Answer from the drawing. Dimensions are ordinates in mm from the lowest x, y and z of the part. Coordinates: 2 decimals unless noted, no trailing zeros. Order: outer loops, then holes, each group sorted by start corner. A loop starts at its lowest first (then second) coordinate and runs counter-clockwise, first axis right, second up. Notation, with made-up numbers: (28, 40.5) - (59, 40.5) arc R5 cw to (59, 47.5) - close; hole circle Ø1 at (-26.5, 27). An arc over 180 degrees is marked (long way). Use CSV: the item, a comma, the result in double quotes. Start each with the question number.
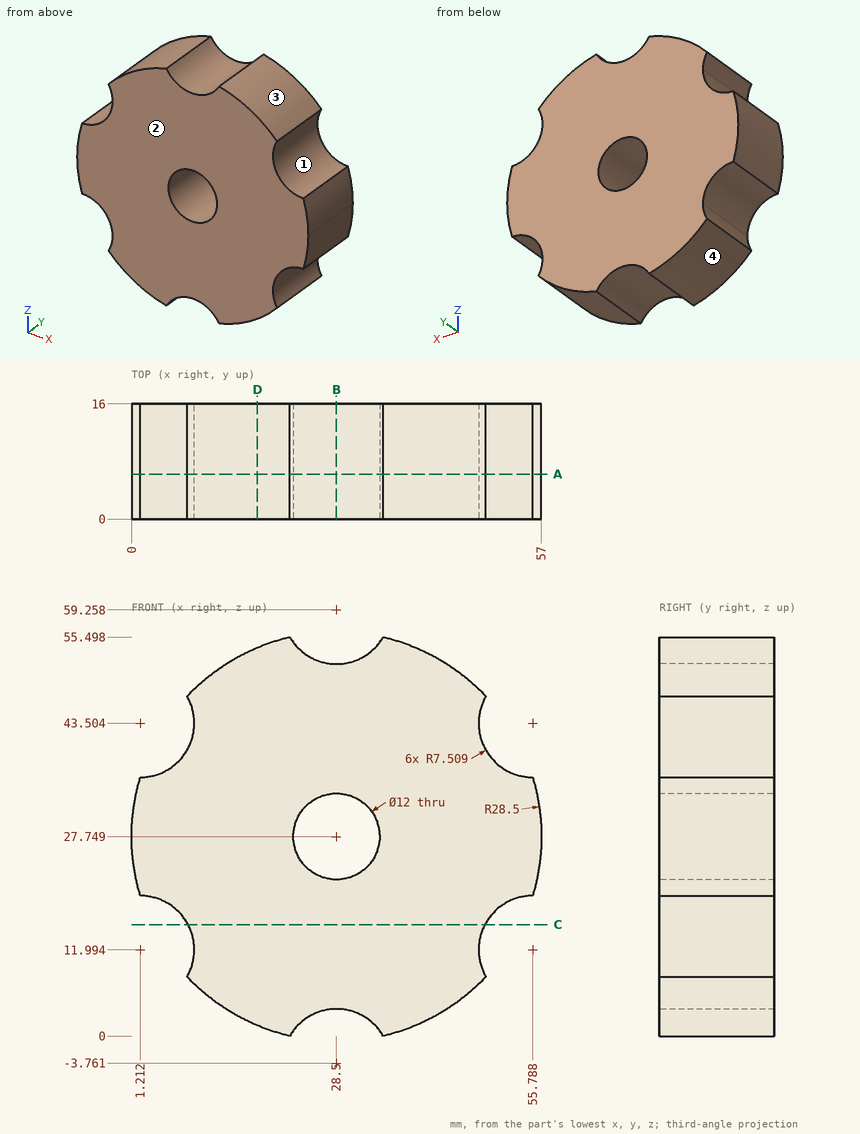
1) Straight lines are drawn through the part: line 1 (X direction, y = 10.75, z = 28) (1 decimal); line 2 (Z direction, x = 23.5, y = 13.25) (1 decimal); line 3 (X direction, y = 4.75, z = 29). For each, find the intervals that lie inside material, in ascending order. Write a range as [from, to].
2) The part is cut by section B-B on x = 28.5. Determine the outline of the cut face in (y, z).
3) The part is cut by section D-D on x = 17.5. Determine the outline of the cut face in (y, z).
4) The part is cut by section C-C on z = 15.5. Determine the outline of the cut face in (x, y), plus the area to 3 significant figures.
5) For a pull along Z with two mould halves and no side action, classify the marked faces 1, 2, 3 and 4 as +Z half, -Z half, draft (parallel to the pull), parting line (faces both ways), or undercut.
6) Flat-ended cylindrical pins translate along their axes: P1, Ø4, axis at y = 10.5, z = 11, coming from the +X side; P2, Ø1, axis at x = 37.5, y = 3.5, coming from the -Z side; P3, Ø1.5, axis at y = 12.5, z = 39, coming from the -X side. Find the tip coordinate at first contact, or state that the pin passes through.
7) The part is cut by section A-A on y = 6.25. Determine the outline of the cut face in (x, z) (1 decimal).
Answer key:
1,line 1,"[0, 22.5], [34.5, 57]"
1,line 2,"[1.8, 24.4], [31.1, 53.7]"
1,line 3,"[0.03, 22.63], [34.37, 56.97]"
2,outline,"(0, 3.75) - (16, 3.75) - (16, 21.75) - (0, 21.75) - close; (0, 33.75) - (16, 33.75) - (16, 51.75) - (0, 51.75) - close"
3,outline,"(0, 1.46) - (16, 1.46) - (16, 54.04) - (0, 54.04) - close"
4,outline,"(7.85, 0) - (49.15, 0) - (49.15, 16) - (7.85, 16) - close"
4,area,"661 mm^2"
5,face 1,"undercut"
5,face 2,"draft"
5,face 3,"+Z half"
5,face 4,"-Z half"
6,P1,"x = 48.9"
6,P2,"z = 0.55"
6,P3,"x = 6.58"
7,outline,"(1.2, 19.5) arc R7.5 cw to (7.7, 8.2) arc R28.5 ccw to (22, 0) arc R7.5 cw to (35, 0) arc R28.5 ccw to (49.3, 8.2) arc R7.5 cw to (55.8, 19.5) arc R28.5 ccw to (55.8, 36) arc R7.5 cw to (49.3, 47.3) arc R28.5 ccw to (35, 55.5) arc R7.5 cw to (22, 55.5) arc R28.5 ccw to (7.7, 47.3) arc R7.5 cw to (1.2, 36) arc R28.5 ccw to start; hole circle Ø12 at (28.5, 27.7)"
